from build123d import *

# Parameters (mm, degrees)
SKETCH1_W                = 259.8
SKETCH1_H                = 349.8
SKETCH1_R                = 101.6
BOSS_EXTRUDE1_DEPTH      = 6.35
M8_CLEARANCE_HOLE1_D     = 8.4
M8_CLEARANCE_HOLE1_DEPTH = 76.2
M8_CLEARANCE_HOLE1_TIP   = 2.5236146


with BuildPart() as part:
    # Sketch1 → Boss-Extrude1 (new body)
    with BuildSketch(Plane.XY):
        with Locations((-129.9, 174.9)):
            Rectangle(SKETCH1_W, SKETCH1_H)
        with Locations((-129.9, 174.9)):
            Circle(SKETCH1_R, mode=Mode.SUBTRACT)
    extrude(amount=BOSS_EXTRUDE1_DEPTH)

    # M8 Clearance Hole1
    with Locations(Plane.XY.offset(6.35)):
        with Locations((-237.3, 327.3), (-22.5, 327.3), (-22.5, 22.5), (-237.3, 22.5)):
            Hole(M8_CLEARANCE_HOLE1_D / 2, depth=M8_CLEARANCE_HOLE1_DEPTH)
            with Locations((0, 0, -(M8_CLEARANCE_HOLE1_DEPTH + M8_CLEARANCE_HOLE1_TIP / 2))):  # 118° drill point
                Cone(0, M8_CLEARANCE_HOLE1_D / 2, M8_CLEARANCE_HOLE1_TIP, mode=Mode.SUBTRACT)


solid = part.part
Source: CAD feature listing. Evaluate the final solid. Frame: model axes, mm. Round coordinates to 2 decimals unless told otherwise and drop trailing zeros. Loops run counter-clockwise (first coordinate to the right, second up) from the corner with the lowest first, then second, coordinate; pieces in that order, holes last.
Q1. Section C-C, the plane z = 4.75. Return loops of the section in (x, y).
Q2. Section D-D, the plane x = -237.3. Return loops of the section in (y, z).
Q3. Section A-A, the plane y = 327.3. Return loops of the section in (x, z), plus the area to 3 significant figures.
Q4. Section B-B, the plane x = -129.9. Return loops of the section in (y, z).
Q5. Ray query, line 1 (Y direction, x = -22.5, z = 3.75); line 2 (X direction, y = 327.3, z = 1.5); line 3 (Y direction, x = -131, z = 1.75). Return the intervals inside material, ascending.
Q6. Mould query, pull axis Y, two halves, no side actions, for faces 1 (the face through (-239.56, 26.04, 3.13)), 2 (the face through (-16, 177, 0)), 3 (the face through (-36.047, 135.987, 3.131)). Classes: pulls with the +Y half, pulls with the -Y half, needs draft (parallel to the pull), parting line crosses it, or undercut.
Q7. First-contact query: P1, Ø5, axis at x = -22.5, y = 327.3, coming from the -Z side. Flat tip, straight axial feed; report the tip coordinate or a pass-through.
Solutions:
1. outline: (-259.8, 0) - (0, 0) - (0, 349.8) - (-259.8, 349.8) - close; hole circle Ø8.4 at (-237.3, 22.5); hole circle Ø8.4 at (-237.3, 327.3); hole circle Ø203.2 at (-129.9, 174.9); hole circle Ø8.4 at (-22.5, 22.5); hole circle Ø8.4 at (-22.5, 327.3)
2. outline: (0, 0) - (18.3, 0) - (18.3, 6.35) - (0, 6.35) - close; (26.7, 0) - (323.1, 0) - (323.1, 6.35) - (26.7, 6.35) - close; (331.5, 0) - (349.8, 0) - (349.8, 6.35) - (331.5, 6.35) - close
3. outline: (-259.8, 0) - (-241.5, 0) - (-241.5, 6.35) - (-259.8, 6.35) - close; (-233.1, 0) - (-26.7, 0) - (-26.7, 6.35) - (-233.1, 6.35) - close; (-18.3, 0) - (0, 0) - (0, 6.35) - (-18.3, 6.35) - close
3. area: 1,540 mm2
4. outline: (0, 0) - (73.3, 0) - (73.3, 6.35) - (0, 6.35) - close; (276.5, 0) - (349.8, 0) - (349.8, 6.35) - (276.5, 6.35) - close
5. line 1: y = 0 to 18.3, 26.7 to 323.1, 331.5 to 349.8
5. line 2: x = -259.8 to -241.5, -233.1 to -26.7, -18.3 to 0
5. line 3: y = 0 to 73.31, 276.49 to 349.8
6. face 1: undercut
6. face 2: needs draft
6. face 3: undercut
7. P1: passes through
